Verification items for the finished model (mm, model axes). Face numbers are marked on the shaded views. Coordinates: 2 decimals unless noted, no trailing zeros. Write each loop counter-clockwise with the first axis right and the second up, starting at its lowest first coordinate (ties: lowest second). Pieces come first, ordered by that corner, then holes. Notation, with made-up numbers: (30.5, 51) -> (48.5, 51) arc R14 ccw to (48.5, 77) -> close; hole circle Ø4 at (18.5, -36.5). An arc over 180 degrees is marked (long way). Answer in a Markdown table with one row per item.
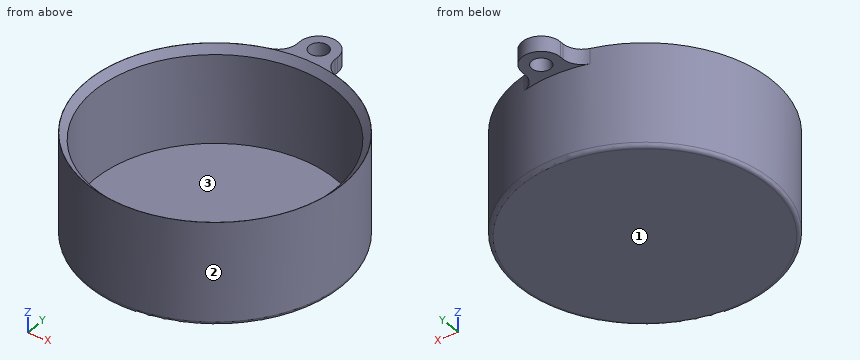
```python
from build123d import *

# Parameters (mm, degrees)
SKETCH_R     = 33.5
PAD_DEPTH    = 27
SKETCH001_R  = 31.65
POCKET_DEPTH = 25
FILLET_R     = 1
CHAMFER_SIZE = 1.8
SKETCH002_R  = 2.5
PAD001_DEPTH = 4
FILLET001_R  = 5
FILLET002_R  = 5


with BuildPart() as part:
    # Sketch → Pad (new body)
    with BuildSketch(Plane.XY):
        Circle(SKETCH_R)
    extrude(amount=PAD_DEPTH)

    # Sketch001 (on Face3 of Pad) → Pocket (cut)
    with BuildSketch(Plane.XY.offset(27)):
        Circle(SKETCH001_R)
    extrude(amount=-POCKET_DEPTH, mode=Mode.SUBTRACT)

    # Fillet
    fillet_edges = [part.edges().sort_by_distance(p)[0] for p in [
        (-33.5, 0, 0),
    ]]
    fillet(fillet_edges, radius=FILLET_R)

    # Chamfer
    chamfer_edges = [part.edges().sort_by_distance(p)[0] for p in [
        (-31.65, 0, 27),
    ]]
    chamfer(chamfer_edges, length=CHAMFER_SIZE)

    # Sketch002 (on Face1 of Chamfer) → Pad001 (join)
    with BuildSketch(Plane.XY.offset(27)):
        with BuildLine():
            Line((-5, 33.124764), (-5, 38.124764))
            ThreePointArc((5, 38.124764), (0, 43.124764), (-5, 38.124764))
            Line((5, 33.124764), (5, 38.124764))
            ThreePointArc((5, 33.124764), (0, 33.5), (-5, 33.124764))
        make_face()
        with Locations((0, 38.124764)):
            Circle(SKETCH002_R, mode=Mode.SUBTRACT)
    extrude(amount=-PAD001_DEPTH)

    # Fillet001
    fillet001_edges = [part.edges().sort_by_distance(p)[0] for p in [
        (-5, 33.124764, 25),
    ]]
    fillet(fillet001_edges, radius=FILLET001_R)

    # Fillet002
    fillet002_edges = [part.edges().sort_by_distance(p)[0] for p in [
        (5, 33.124764, 25),
    ]]
    fillet(fillet002_edges, radius=FILLET002_R)


solid = part.part
```
1. Sectioned sample at B-B, the plane y = 0. Record the cut outline in (x, z), and give its area (3 significant figures).
Findings below:
| item | result |
|---|---|
| outline | (-33.5, 1) arc R1 ccw to (-32.5, 0) -> (32.5, 0) arc R1 ccw to (33.5, 1) -> (33.5, 27) -> (33.45, 27) -> (31.65, 25.2) -> (31.65, 2) -> (-31.65, 2) -> (-31.65, 25.2) -> (-33.45, 27) -> (-33.5, 27) -> close |
| area | 223 mm² |
2. Go/stop test with flat-tipped pins: pin 1 (12 mm diameter, centred on x = -6.5, z = 22.5, fed in from -Y); pin 2 (4 mm diameter, centred on x = 22.5, z = 21, fed in from +Y); pin 3 (2 mm diameter, centred on x = -24.5, z = 4.5, fed in from -Y); pin 4 (4 mm diameter, centred on x = 0, y = 38.12, fed in from -Z). Record where each tip stops, or that it passes through.
Findings below:
| item | result |
|---|---|
| pin 1 | stops at y = -33.5 |
| pin 2 | stops at y = 26.5 |
| pin 3 | stops at y = -23.87 |
| pin 4 | passes through |
3. Sectioned sample at C-C, the plane z = 12. Record the cut outline in (x, y).
Findings below:
| item | result |
|---|---|
| outline | circle Ø67 at (0, 0); hole circle Ø63.3 at (0, 0) |
4. Sectioned sample at A-A, the plane x = 0. Record the cut outline in (y, z).
Findings below:
| item | result |
|---|---|
| outline | (-33.5, 1) arc R1 ccw to (-32.5, 0) -> (32.5, 0) arc R1 ccw to (33.5, 1) -> (33.5, 23) -> (35.62, 23) -> (35.62, 27) -> (33.45, 27) -> (31.65, 25.2) -> (31.65, 2) -> (-31.65, 2) -> (-31.65, 25.2) -> (-33.45, 27) -> (-33.5, 27) -> close; (40.62, 23) -> (43.12, 23) -> (43.12, 27) -> (40.62, 27) -> close |
5. Material ranges on probe 1 along Y at (x, z) = (0, 24.15); probe 2 along Y at (x, z) = (0, 16.25); probe 3 along Y at (x, z) = (0, 25.25), recorded low to high. Write a range as from..to.
Findings below:
| item | result |
|---|---|
| probe 1 | y = -33.5..-31.65, 31.65..35.62, 40.62..43.12 |
| probe 2 | y = -33.5..-31.65, 31.65..33.5 |
| probe 3 | y = -33.5..-31.7, 31.7..35.62, 40.62..43.12 |
6. Release check for a two-part mould opening along X. For the marked faces 1, 2 and 3 record: released by +X, released by -X, zero draft, split by the parting line, or undercut.
Findings below:
| item | result |
|---|---|
| face 1 | zero draft |
| face 2 | split by the parting line |
| face 3 | undercut |
